```python
from build123d import *

# Parameters (mm, degrees)
F0_R     = 2.15265
F0_R_2   = 5.5
F1_DEPTH = 3.175


with BuildPart() as f1:
    # F0 (on Top) → F1 (new body)
    with BuildSketch(Plane.XY):
        with BuildLine():
            Line((18.280792, -11.672377), (7.203258, 4.834118))
            ThreePointArc((7.203258, 4.834118), (0, 8.675), (-7.203258, 4.834118))
            Line((-7.203258, 4.834118), (-18.280792, -11.672377))
            ThreePointArc((-18.280792, -11.672377), (-18.528679, -16.567053), (-14.326265, -19.088765))
            Line((-14.326265, -19.088765), (14.326265, -19.088765))
            ThreePointArc((14.326265, -19.088765), (18.528679, -16.567053), (18.280792, -11.672377))
        make_face()
        with Locations((-14.326265, -14.326265)):
            Circle(F0_R, mode=Mode.SUBTRACT)
        with Locations((14.326265, -14.326265)):
            Circle(F0_R, mode=Mode.SUBTRACT)
        Circle(F0_R_2, mode=Mode.SUBTRACT)
    extrude(amount=F1_DEPTH)


solid = f1.part
```
Verification items for the finished model (mm, model axes). Give positions to 0.01 mm unless a question says otherwise; leave off trailing zeros. Order: outer loops, then holes, each group sorted by start corner. A loop starts at its lowest first (then second) coordinate and runs counter-clockwise, first axis right, second up. Notation, with made-up numbers: M 12.5,53 L 53.5,53 A33 cw 53.5,85 Z; hole C 67,29.5 d8. An arc over 180 degrees is marked long. Return JSON: item names as keys, results as strings. Group by question number.
1) Section check B-B on z = 2.45. Give the number of separate pieces and of enclosed holes in the cut face, and give its area (3 significant figures).
2) Scan lines: line 1 (X direction, y = -15.5, z = 0.2); line 2 (X direction, y = -14, z = 1.5); line 3 (Y direction, x = 2, z = 2.7). Record each from-to range of solid material in increasing order.
3) Mould release check, pull along Y, two halves, no side actions. Record for faces 1 (the face through (-12.273, -13.68, 1.565)), 2 (the face through (16.315, -15.151, 1.565)), 3 (the face through (12.82, -3.535, 1.565)), 4 (the face through (18.494, -16.63, 1.565)): pulls with the +Y half, pulls with the -Y half, needs draft (parallel to the pull), parting line crosses it, or undercut.
4) Section check C-C on y = -1. Record the cut outline in (x, z) (3 decimals), and give its area (3 significant figures).
5) Go/stop test with flat-tipped pins: pin 1 Ø1 at (y, z) = (-13.5, 2.5) entering from -X; pin 2 Ø1.5 at (y, z) = (5.5, 2) entering from +X; pin 3 Ø1.5 at (y, z) = (-10.5, 2.5) entering from +X. Record where each tip stops, or that it passes through.
6) Section check A-A on x = 0. Record the cut outline in (y, z) (3 decimals).
7) Section check D-D on y = -8.75. Record the cut outline in (x, z) (3 decimals).
Answer block:
{
 "1": {"separate pieces": "1", "enclosed holes": "3", "area": "607 mm^2"},
 "2": {"line 1": "x = -18.94 to -16.13, -12.52 to 12.52, 16.13 to 18.94", "line 2": "x = -19.08 to -16.45, -12.2 to 12.2, 16.45 to 19.08", "line 3": "y = -19.09 to -5.12, 5.12 to 8.44"},
 "3": {"face 1": "undercut", "face 2": "undercut", "face 3": "pulls with the +Y half", "face 4": "parting line crosses it"},
 "4": {"outline": "M -11.119,0 L -5.408,0 L -5.408,3.175 L -11.119,3.175 Z; M 5.408,0 L 11.119,0 L 11.119,3.175 L 5.408,3.175 Z", "area": "36.3 mm^2"},
 "5": {"pin 1": "stops at x = -19.08", "pin 2": "stops at x = 7.26", "pin 3": "stops at x = 18"},
 "6": {"outline": "M -19.089,0 L -5.5,0 L -5.5,3.175 L -19.089,3.175 Z; M 5.5,0 L 8.675,0 L 8.675,3.175 L 5.5,3.175 Z"},
 "7": {"outline": "M -16.32,0 L 16.32,0 L 16.32,3.175 L -16.32,3.175 Z"}
}
